Could you check a few things on this model? Use its own coordinates, in mm. Face numbers are marked on the shaded views. Coordinates: 2 decimals unless noted, no trailing zeros. Loops run counter-clockwise (first coordinate to the right, second up) from the corner with the lowest first, then second, coordinate; pieces in that order, holes last. Notation, with made-up numbers: (74.25, 83) - (84.25, 83) arc R18 ccw to (84.25, 115) - close; hole circle Ø3 at (10, 69). An arc over 180 degrees is marked (long way). Put each result on its own line as item: value. Start each with the question number.
```python
from build123d import *

# Parameters (mm, degrees)
F1_DEPTH      = 177.8
F1_DEPTH_BACK = 76.2
F2_R          = 0.508
F4_DEPTH      = 14.6291181898
F4_DEPTH_BACK = 14.6291181898
F6_DEPTH      = 25.4737621135
F8_DEPTH      = 14.6291181898
F8_DEPTH_BACK = 14.6291181898
F9_R          = 4.7625


with BuildPart() as f1:
    # F0 (on Front) → F1 (new body, two sides)
    with BuildSketch(Plane.XZ) as f1_sk:
        Polygon((0, 25.9807621135), (-15, 0), (15, 0), align=None)
        Polygon((-12.4019237886, 1.5), (0, 22.9807621135), (12.4019237886, 1.5), align=None, mode=Mode.SUBTRACT)
    extrude(amount=F1_DEPTH)
    extrude(f1_sk.sketch, amount=-F1_DEPTH_BACK)

    # F2
    f2_edges = [f1.edges().sort_by_distance(p)[0] for p in [
        (0, -50.8, 25.980762),
        (15, -50.8, 0),
        (-15, -50.8, 0),
        (-12.401924, -50.8, 1.5),
        (0, -50.8, 22.980762),
        (12.401924, -50.8, 1.5),
    ]]
    fillet(f2_edges, radius=F2_R)

    # F3 (on Right) → F4 (cut, two sides)
    with BuildSketch(Plane.YZ) as f4_sk:
        with BuildLine():
            Line((-8.6871078238, 16.7701914907), (-8.6706578732, 12.6613909379))
            Line((-8.6706578732, 12.6613909379), (0, 6.2201358425))
            Line((0, 6.2201358425), (8.6693109221, 12.6603903153))
            Line((8.6693109221, 12.6603903153), (8.6693109221, 16.7701914907))
            ThreePointArc((8.6693109221, 16.7701914907), (-0.0088984509, 22.3225436807), (-8.6871078238, 16.7701914907))
        make_face()
    extrude(amount=-F4_DEPTH, mode=Mode.SUBTRACT)
    extrude(f4_sk.sketch, amount=F4_DEPTH_BACK, mode=Mode.SUBTRACT)

    # F5 (on Top) → F6 (cut, through all)
    with BuildSketch(Plane.XY):
        with BuildLine():
            Line((-5.0927, -172.72), (-5.0927, -165.1))
            ThreePointArc((-5.0927, -165.1), (-6.35, -163.8427), (-7.6073, -165.1))
            Line((-7.6073, -165.1), (-7.6073, -172.72))
            ThreePointArc((-7.6073, -172.72), (-6.35, -173.9773), (-5.0927, -172.72))
        make_face()
        with BuildLine():
            ThreePointArc((7.6073, -165.1), (6.35, -163.8427), (5.0927, -165.1))
            Line((5.0927, -165.1), (5.0927, -172.72))
            ThreePointArc((5.0927, -172.72), (6.35, -173.9773), (7.6073, -172.72))
            Line((7.6073, -172.72), (7.6073, -165.1))
        make_face()
    extrude(amount=F6_DEPTH, mode=Mode.SUBTRACT)

    # F7 (on Right) → F8 (cut, two sides)
    with BuildSketch(Plane.YZ) as f8_sk:
        Polygon((-204.1564583778, 33.782), (-205.74, 2.032), (-154.94, 2.032), (-136.6091289532, 33.782), align=None)
    extrude(amount=-F8_DEPTH, mode=Mode.SUBTRACT)
    extrude(f8_sk.sketch, amount=F8_DEPTH_BACK, mode=Mode.SUBTRACT)

    # F9
    f9_edges = [f1.edges().sort_by_distance(p)[0] for p in [
        (12.928149, -154.94, 2.032),
        (-12.928149, -154.94, 2.032),
    ]]
    fillet(f9_edges, radius=F9_R)


solid = f1.part
```
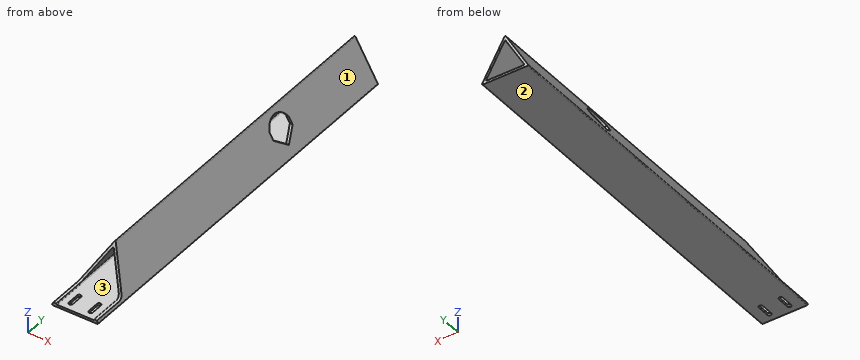
(1) If we mould it in two halves opening along Z, with no side actions, what happens to the marked faces 1, 2 and 3? For each: pulls with the +Z half, pulls with the -Z half, needs draft (parallel to the pull), parting line crosses it, or undercut.
(2) I need wall thicknesses on L1, parallel to Z at x = 2, y = -158.5; L2, parallel to X at y = 64.5, z = 17.75; L3, parallel to Z at x = -5.5, y = -30.5. Which ranges of each line are inside material? Lowest first, please. Write a range as [from, to].
(3) For pin 1 Ø0.8 at (y, z) = (-169, 1) entering from -X; pin 2 Ø4 at (y, z) = (-133.5, 11) entering from -X; pin 3 Ø12 at (x, z) = (-5, 18) entering from +Y; pin 4 Ø2 at (x, z) = (5, 14) entering from -Y, each with a flat end and sliding along its axis, tell me the tip position at first contact or that it passes through.
(4) I want a section at A-A on y = -119.5. List the corners of the cut face in (x, z) for me, and give its area (3 significant figures).
Answer sheet:
1. face 1: pulls with the +Z half
1. face 2: pulls with the -Z half
1. face 3: undercut
2. L1: z = [0, 1.5]
2. L2: x = [-4.75, -3.02], [3.02, 4.75]
2. L3: z = [0, 1.5], [13.45, 16.45]
3. pin 1: stops at x = -14.62
3. pin 2: stops at x = -9.8
3. pin 3: stops at y = 76.2
3. pin 4: stops at y = -148.48
4. outline: (-14.56, 0.76) arc R0.51 ccw to (-14.12, 0) - (14.12, 0) arc R0.51 ccw to (14.56, 0.76) - (0.44, 25.22) arc R0.51 ccw to (-0.44, 25.22) - close; hole (-11.96, 2.26) arc R0.51 ccw to (-11.52, 1.5) - (11.52, 1.5) arc R0.51 ccw to (11.96, 2.26) - (0.44, 22.22) arc R0.51 ccw to (-0.44, 22.22) - close
4. area: 123 mm^2
